from build123d import *


with BuildPart() as part:
    # Sketch1 → Revolve1 (revolve)
    with BuildSketch(Plane(origin=(0, 0, 0), x_dir=(0, 0, -1), z_dir=(1, 0, 0))):
        with BuildLine():
            Line((11, -10), (11, 10))
            Line((11, 10), (16, 10))
            Line((16, 10), (16, 5))
            ThreePointArc((16, 5), (16.585786438, 3.585786438), (18, 3))
            Line((18, 3), (45, 3))
            ThreePointArc((45, 3), (46.414213562, 3.585786438), (47, 5))
            Line((47, 5), (47, 13))
            Line((47, 13), (50, 13))
            Line((50, 13), (50, -13))
            Line((50, -13), (47, -13))
            Line((47, -13), (47, -5))
            ThreePointArc((47, -5), (46.414213562, -3.585786438), (45, -3))
            Line((45, -3), (18, -3))
            ThreePointArc((18, -3), (16.585786438, -3.585786438), (16, -5))
            Line((16, -5), (16, -10))
            Line((16, -10), (11, -10))
        make_face()
    revolve(axis=Axis((0, 0, 0), (0, 1, 0)))


solid = part.part
Geometry: final body of the model. Coordinates: model frame, mm. A direction names the side the tool comes from. Round coordinates to 2 decimals unless told otherwise and drop trailing zeros. Loops run counter-clockwise (first coordinate to the right, second up) from the corner with the lowest first, then second, coordinate; pieces in that order, holes last. Notation, with made-up numbers: M 64,72 L 91,72 A20 cw 91,90 Z; hole C 72.5,-3 d2. An arc over 180 degrees is marked long. Put each result on its own line as item: value. Start each with the question number.
(1) Set-up query: faces 4 (the face through (19, -3, 1)), 5 (the face through (10.74, 0.14, 2.38)), 6 (the face through (-11, 10, 3)). Return all of +Z, -Z, +X, -X, +Y, -Y with unobstructed straight access to the full face (end or side cutting, diameter ignored); none if empty.
(2) Section query C-C (y = 11.75). Return loops of the section in (x, z).
(3) Material intervals for line 1 along Z through (x, y) = (0, -7); line 2 along X through (y, z) = (5, -10); line 3 along Z through (x, y) = (6.5, 5.25), sorted ascending. Write a range as [from, to].
(4) Contact query for flat-ended pins moving along their axis: pin 1 Ø1.5 at (x, y) = (-32, 0) entering from +Z; pin 2 Ø2 at (x, z) = (18, 10) entering from -Y; pin 3 Ø2 at (y, z) = (1, 28) entering from -X. Output: stop coordinate, or through.
(5) Draft query along X for faces 1 (the face through (-11, -10, -3)), 2 (the face through (33, 13, -34)), 3 (the face through (-15.02, -0.18, -47.69)). Return one class per face: +X half, -X half, draft (parallel to the pull), parting line (faces both ways), or undercut.
Findings below:
1. face 4: -Y
1. face 5: +Y, -Y
1. face 6: +Y
2. outline: C 0,0 d100; hole C 0,0 d94
3. line 1: z = [-50, -47], [-16, -11], [11, 16], [47, 50]
3. line 2: x = [-48.99, -45.92], [-12.49, -4.58], [4.58, 12.49], [45.92, 48.99]
3. line 3: z = [-49.58, -46.55], [-14.62, -8.87], [8.87, 14.62], [46.55, 49.58]
4. pin 1: stops at z = 39.03
4. pin 2: stops at y = -3
4. pin 3: stops at x = -42.08
5. face 1: undercut
5. face 2: draft
5. face 3: parting line
